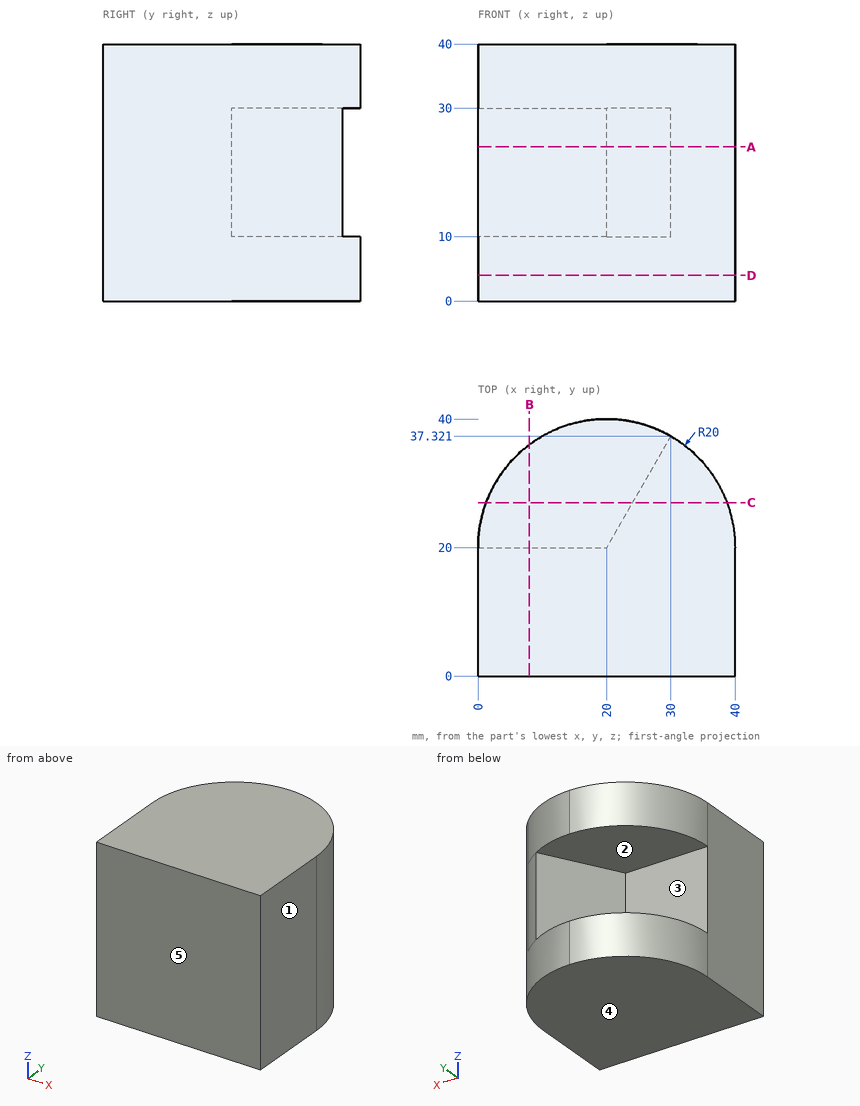
Could you check a few things on this drawing? It's one solid part, dimensions in mm from its lowest x, y, z. A direction names the side the tool comes from. Coordinates: 2 decimals unless noted, no trailing zeros. Order: outer loops, then holes, each group sorted by start corner. A loop starts at its lowest first (then second) coordinate and runs counter-clockwise, first axis right, second up. Notation, with made-up numbers: (66, 38) - (74, 38) arc R13 ccw to (74, 50) - close; hole circle Ø3 at (3, -9). An arc over 180 degrees is marked (long way). Answer as a JSON object with one key per item and string values. Group by question number.
Q1. We'd pull the mould along Z, two halves only. Please class the marked faces 3, 4 and 5: +Z half, -Z half, draft (parallel to the pull), parting line (faces both ways), or undercut.
Q2. Imagine slicing it at B-B (x = 8). Please give me the cut outline in (y, z), and give its area (3 significant figures).
Q3. On a 3-axis mill with a long thin cutter (end or side, diameter ignored), from which of +Z, -Z, +X, -X, +Y, -Y can I reach the whole of each face in a straight line? I mean the marked faces 1 and 2. Say none if no direction works.
Q4. I need wall thicknesses on line 1 (Z direction, x = 9, y = 27.5); line 2 (Y direction, x = 19, z = 29); line 3 (Y direction, x = 10, z = 36.5). Which ranges of each line are inside material? Lowest first, please. Write a range as from..to.
Q5. Imagine slicing it at D-D (z = 4). Please give me the cut outline in (x, y), and give its area (3 significant figures).
Q6. Will these pins go through, and if not, where does the flat tip stop? P1, Ø5, axis at x = 15.5, y = 30.5, coming from the -Z side; P2, Ø12, axis at y = 28.5, z = 15.5, coming from the +X side; P3, Ø6, axis at x = 6, z = 15, coming from the +Y side; P4, Ø2, axis at y = 35.5, z = 34.5, coming from the +X side (1 decimal).
Q7. Imagine slicing it at A-A (z = 24). Please give me the cut outline in (x, y).
Q8. Imagine slicing it at C-C (y = 27). Please give me the cut outline in (x, z) (1 decimal).
Determined:
{
 "1": {"face 3": "undercut", "face 4": "-Z half", "face 5": "draft"},
 "2": {"outline": "(0, 0) - (36, 0) - (36, 10) - (20, 10) - (20, 30) - (36, 30) - (36, 40) - (0, 40) - close", "area": "1,120 mm2"},
 "3": {"face 1": "+Z, -Z, +X, +Y, -Y", "face 2": "-X, +Y"},
 "4": {"line 1": "z = 0..10, 30..40", "line 2": "y = 0..20", "line 3": "y = 0..37.32"},
 "5": {"outline": "(0, 0) - (40, 0) - (40, 20) arc R20 ccw to (0, 20) - close", "area": "1,430 mm2"},
 "6": {"P1": "stops at z = 0", "P2": "stops at x = 39.84", "P3": "stops at y = 20", "P4": "stops at x = 33.8"},
 "7": {"outline": "(0, 0) - (40, 0) - (40, 20) arc R20 ccw to (30, 37.32) - (20, 20) - (0, 20) - close"},
 "8": {"outline": "(1.3, 0) - (38.7, 0) - (38.7, 40) - (1.3, 40) - (1.3, 30) - (24, 30) - (24, 10) - (1.3, 10) - close"}
}
